```python
from build123d import *

# Parameters (mm, degrees)
SKETCH1_R           = 13
SKETCH1_R_2         = 2.65
BOSS_EXTRUDE1_DEPTH = 3
SKETCH2_W           = 1.2
SKETCH2_H           = 3.758494417
CUT_EXTRUDE1_DEPTH  = 19.62793601
CIRPATTERN1_COUNT   = 20


with BuildPart() as part:
    # Sketch1 → Boss-Extrude1 (new body)
    # profile 1 of 3: a face of its own
    with BuildSketch(Plane.XY):
        Circle(SKETCH1_R)
        Circle(SKETCH1_R_2, mode=Mode.SUBTRACT)
    # profile 2 of 3: a face of its own
    with BuildSketch(Plane.XY):
        with BuildLine():
            Line((-1.75, -1.989974874), (-1.75, 1.989974874))
            ThreePointArc((-1.75, 1.989974874), (-2.65, 0), (-1.75, -1.989974874))
        make_face()
    # profile 3 of 3: a face of its own
    with BuildSketch(Plane.XY):
        with BuildLine():
            ThreePointArc((2.65, 0), (2.414539294, 1.092016483), (1.75, 1.989974874))
            Line((1.75, 1.989974874), (1.75, -1.989974874))
            ThreePointArc((1.75, -1.989974874), (2.414539294, -1.092016483), (2.65, 0))
        make_face()
    extrude(amount=BOSS_EXTRUDE1_DEPTH)

    # Sketch2 → Cut-Extrude1 (cut, through all)
    with BuildSketch(Plane.XY.offset(3)):
        with Locations((0, 9.104376966)):
            Rectangle(SKETCH2_W, SKETCH2_H)
    cut_extrude1 = extrude(amount=-CUT_EXTRUDE1_DEPTH, mode=Mode.SUBTRACT)

    # CirPattern1: Cut-Extrude1 ×20 about axis
    cirpattern1_axis = Axis((0, 0, 0), (0, 0, 1))
    for i in range(1, CIRPATTERN1_COUNT):
        add(cut_extrude1.rotate(cirpattern1_axis, i * 360 / CIRPATTERN1_COUNT), mode=Mode.SUBTRACT)


solid = part.part
```
Geometry: final body of the model. Coordinates: model frame, mm. Coordinates: 2 decimals unless noted, no trailing zeros. Order: outer loops, then holes, each group sorted by start corner. A loop starts at its lowest first (then second) coordinate and runs counter-clockwise, first axis right, second up. Notation, with made-up numbers: (61, -15.5) -> (100, -15.5) arc R25 ccw to (100, -3.5) -> close; hole circle Ø4 at (29.25, 47). An arc over 180 degrees is marked (long way). Write item = value, one per line.
(1) Cut plane B-B on y = 0. Return loops of the section in (x, z), plus the area to 3 significant figures.
Solved:
outline = (-13, 0) -> (-10.98, 0) -> (-10.98, 3) -> (-13, 3) -> close; (-7.23, 0) -> (-1.75, 0) -> (-1.75, 3) -> (-7.23, 3) -> close; (1.75, 0) -> (7.23, 0) -> (7.23, 3) -> (1.75, 3) -> close; (10.98, 0) -> (13, 0) -> (13, 3) -> (10.98, 3) -> close
area = 44.9 mm²
(2) Pull-direction query (Y, two-part tool) for faces 1 (the flat face through (0, -3, 3)), 2 (the flat face through (-10.449, 3.386, 1.521)); classes: pulls with the +Y half, pulls with the -Y half, needs draft (parallel to the pull), parting line crosses it, or undercut.
Solved:
face_1 = needs draft
face_2 = undercut
(3) Cut plane C-C on z = 1.5. Count the separate pieces of the cut face and the enclosed holes in it, plus the area to 3 significant figures.
Solved:
separate_pieces = 1
enclosed_holes = 21
area = 424 mm²
(4) Line query: line 1 (X direction, y = -10, z = 2.3); line 2 (Y direction, x = 8, z = 2.25); line 3 (Y direction, x = -6, z = 1.7). Output: solid intervals per line, ascending.
Solved:
line_1 = -8.31 to -3.88, -2.62 to -0.6, 0.6 to 2.62, 3.88 to 8.31
line_2 = -10.25 to -6.55, -5.07 to -3.23, -1.97 to -0.6, 0.6 to 1.97, 3.23 to 5.07, 6.55 to 10.25
line_3 = -11.53 to -9.22, -7.24 to -5.1, -4.03 to 4.03, 5.1 to 7.24, 9.22 to 11.53
(5) Pin query (flat end, axial travel): pin 1 Ø1 at (y, z) = (-4, 1.5) entering from +X; pin 2 Ø5 at (x, y) = (-6, -9) entering from -Z; pin 3 Ø1.5 at (y, z) = (4.5, 1) entering from -X; pin 4 Ø0.9 at (x, z) = (-8, 1.5) entering from -Y. Return the tip coordinate at first contact, or that it passes through.
Solved:
pin_1 = 12.52
pin_2 = 0
pin_3 = -12.45
pin_4 = -10.58
(6) Cut plane A-A on x = 0. Return loops of the section in (y, z).
Solved:
outline = (-13, 0) -> (-10.98, 0) -> (-10.98, 3) -> (-13, 3) -> close; (-7.23, 0) -> (-2.65, 0) -> (-2.65, 3) -> (-7.23, 3) -> close; (2.65, 0) -> (7.23, 0) -> (7.23, 3) -> (2.65, 3) -> close; (10.98, 0) -> (13, 0) -> (13, 3) -> (10.98, 3) -> close
